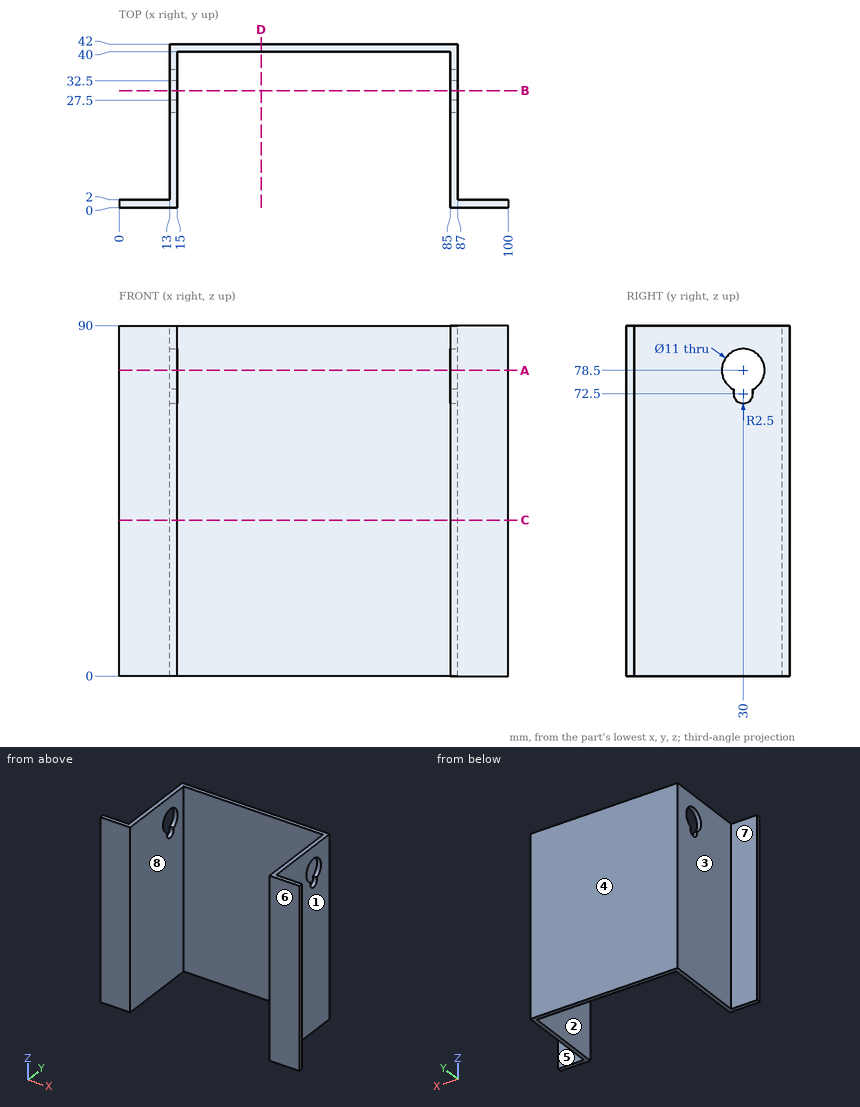
Source: three-view drawing plus pictorial views. Frame: mm from the lowest corner of the part. A direction names the side the tool comes from. Give positions to 0.01 mm unless a question says otherwise; leave off trailing zeros. Loops run counter-clockwise (first coordinate to the right, second up) from the corner with the lowest first, then second, coordinate; pieces in that order, holes last. Notation, with made-up numbers: (-14, 44.5) -> (3, 44.5) arc R18 ccw to (3, 55.5) -> close; hole circle Ø5 at (70, 77.5). An arc over 180 degrees is marked (long way). Put each result on its own line as item: value. Start each with the question number.
1) Cut plane C-C (z = 40). Return loops of the section in (x, y), then the cut area to 3 significant figures.
2) Cut plane A-A (z = 78.5). Return loops of the section in (x, y).
3) Cut plane D-D (x = 36.5). Return loops of the section in (y, z).
4) Draft query along X for the marked faces 1, 2, 3 and 4. Return one class per face: released by +X, released by -X, zero draft, split by the parting line, or undercut.
5) Reachability of the marked faces 5, 6, 7 and 8 from +Z, -Z, +X, -X, +Y, -Y: full face, straight path, thin tool, end or side. Return the list, or none.
6) Contact query for flat-ended pins moving along their axis: P1, Ø10, axis at x = 52, z = 15, coming from the -Y side; P2, Ø6.5, axis at y = 30, z = 78.5, coming from the -X side; P3, Ø12, axis at y = 32, z = 79.5, coming from the +X side; P4, Ø12, axis at y = 26, z = 60, coming from the -X side. Output: stop coordinate, or through.
7) Material intervals for probe 1 along X at (y, z) = (13, 38); probe 2 along Y at (x, z) = (86, 78); probe 3 along Y at (x, z) = (35.5, 70.5), sorted ascending.
8) Cut plane B-B (y = 30). Return loops of the section in (x, z), then the cut area to 3 significant figures.
Results are:
1. outline: (0, 0) -> (15, 0) -> (15, 40) -> (85, 40) -> (85, 0) -> (100, 0) -> (100, 2) -> (87, 2) -> (87, 42) -> (13, 42) -> (13, 2) -> (0, 2) -> close
1. area: 360 mm2
2. outline: (0, 0) -> (15, 0) -> (15, 24.5) -> (13, 24.5) -> (13, 2) -> (0, 2) -> close; (13, 35.5) -> (15, 35.5) -> (15, 40) -> (85, 40) -> (85, 35.5) -> (87, 35.5) -> (87, 42) -> (13, 42) -> close; (85, 0) -> (100, 0) -> (100, 2) -> (87, 2) -> (87, 24.5) -> (85, 24.5) -> close
3. outline: (40, 0) -> (42, 0) -> (42, 90) -> (40, 90) -> close
4. face 1: released by +X
4. face 2: undercut
4. face 3: released by -X
4. face 4: zero draft
5. face 5: +Z, -Z, +X, +Y
5. face 6: +Z, -Z, +X, -X, -Y
5. face 7: +Z, -Z, -X, +Y
5. face 8: +Z, -Z, -Y
6. P1: stops at y = 40
6. P2: passes through
6. P3: stops at x = 87
6. P4: stops at x = 13
7. probe 1: x = 13 to 15, 85 to 87
7. probe 2: y = 0 to 24.52, 35.48 to 42
7. probe 3: y = 40 to 42
8. outline: (13, 0) -> (15, 0) -> (15, 70) -> (13, 70) -> close; (13, 84) -> (15, 84) -> (15, 90) -> (13, 90) -> close; (85, 0) -> (87, 0) -> (87, 70) -> (85, 70) -> close; (85, 84) -> (87, 84) -> (87, 90) -> (85, 90) -> close
8. area: 304 mm2
